from build123d import *

# Parameters (mm, degrees)
BOSS_EXTRUDE1_DEPTH            = 3
SKETCH2_R                      = 2
CUT_EXTRUDE1_DEPTH             = 3
CHAMFER1_SIZE                  = 0.5
LPATTERN1_COUNT                = 14
LPATTERN1_PITCH                = 50
CHAMFER1_OF_LPATTERN1_SIZE     = 0.5
LPATTERN1_COL_COUNT            = 14
LPATTERN1_COL_PITCH            = 50
CHAMFER1_OF_LPATTERN1_COL_SIZE = 0.5
FILLET1_R                      = 1
SKETCH3_R                      = 2.25
CUT_EXTRUDE2_DEPTH             = 10
CHAMFER2_SIZE                  = 0.5
CHAMFER2_OF_MIRROR1_SIZE       = 0.5


with BuildPart() as part:
    # Sketch1 → Boss-Extrude1 (new body)
    with BuildSketch(Plane(origin=(0, 0, 0), x_dir=(0, 0, -1), z_dir=(1, 0, 0))):
        Polygon((-706, 30), (-706, -5), (-671, -5), (-671, -30), (671, -30), (671, -5), (706, -5), (706, 30), align=None)
    extrude(amount=BOSS_EXTRUDE1_DEPTH)

    # Sketch2 → Cut-Extrude1 (cut)
    with BuildSketch(Plane(origin=(3, 0, 0), x_dir=(0, 0, -1), z_dir=(1, 0, 0))):
        with Locations((0, -25)):
            Circle(SKETCH2_R)
    cut_extrude1 = extrude(amount=-CUT_EXTRUDE1_DEPTH, mode=Mode.SUBTRACT)

    # Chamfer1
    chamfer1_edges = [part.edges().sort_by_distance(p)[0] for p in [
        (3, -25, 2),
    ]]
    chamfer(chamfer1_edges, length=CHAMFER1_SIZE)

    # LPattern1: Cut-Extrude1 ×14
    with Locations(*[(0, 0, i * LPATTERN1_PITCH) for i in range(1, LPATTERN1_COUNT)]):
        add(cut_extrude1, mode=Mode.SUBTRACT)

    # Chamfer1 of LPattern1
    chamfer1_of_lpattern1_edges = [part.edges().sort_by_distance(p)[0] for p in [
        (3, -25, 52),
        (3, -25, 102),
        (3, -25, 152),
        (3, -25, 202),
        (3, -25, 252),
        (3, -25, 302),
        (3, -25, 352),
        (3, -25, 402),
        (3, -25, 452),
        (3, -25, 502),
        (3, -25, 552),
        (3, -25, 602),
        (3, -25, 652),
    ]]
    chamfer(chamfer1_of_lpattern1_edges, length=CHAMFER1_OF_LPATTERN1_SIZE)

    # LPattern1 col: Cut-Extrude1 ×14
    with Locations(*[(0, 0, -i * LPATTERN1_COL_PITCH) for i in range(1, LPATTERN1_COL_COUNT)]):
        add(cut_extrude1, mode=Mode.SUBTRACT)

    # Chamfer1 of LPattern1 col
    chamfer1_of_lpattern1_col_edges = [part.edges().sort_by_distance(p)[0] for p in [
        (3, -25, -48),
        (3, -25, -98),
        (3, -25, -148),
        (3, -25, -198),
        (3, -25, -248),
        (3, -25, -298),
        (3, -25, -348),
        (3, -25, -398),
        (3, -25, -448),
        (3, -25, -498),
        (3, -25, -548),
        (3, -25, -598),
        (3, -25, -648),
    ]]
    chamfer(chamfer1_of_lpattern1_col_edges, length=CHAMFER1_OF_LPATTERN1_COL_SIZE)

    # Fillet1
    fillet1_edges = [part.edges().sort_by_distance(p)[0] for p in [
        (1.5, -5, -706),
        (1.5, -30, -671),
        (1.5, -30, 671),
        (1.5, -5, 706),
        (1.5, 30, 706),
        (1.5, 30, -706),
    ]]
    fillet(fillet1_edges, radius=FILLET1_R)

    # Sketch3 → Cut-Extrude2 (cut)
    with BuildSketch(Plane(origin=(3, 0, 0), x_dir=(0, 0, -1), z_dir=(1, 0, 0))):
        with Locations((687, 12)):
            Circle(SKETCH3_R)
    cut_extrude2 = extrude(amount=-CUT_EXTRUDE2_DEPTH, mode=Mode.SUBTRACT)

    # Chamfer2
    chamfer2_edges = [part.edges().sort_by_distance(p)[0] for p in [
        (3, 12, -684.75),
    ]]
    chamfer(chamfer2_edges, length=CHAMFER2_SIZE)

    # Mirror1: Cut-Extrude2 across plane
    add(cut_extrude2.mirror(Plane.XY), mode=Mode.SUBTRACT)

    # Chamfer2 of Mirror1
    chamfer2_of_mirror1_edges = [part.edges().sort_by_distance(p)[0] for p in [
        (3, 12, 684.75),
    ]]
    chamfer(chamfer2_of_mirror1_edges, length=CHAMFER2_OF_MIRROR1_SIZE)


solid = part.part
Source: CAD feature listing. Evaluate the final solid. Frame: model axes, mm. Round coordinates to 2 decimals unless told otherwise and drop trailing zeros.
Q1. Ray query, line 1 (Z direction, x = 2.5, y = 13); line 2 (Y direction, x = 1.5, z = 687); line 3 (Y direction, x = 1.25, z = 300). Return the intervals inside material, ascending.
Q2. Section A-A, the plane x = 1.5. State how many separate pieces and enclosed holes the cut face has, plus the area to 3 significant figures.
Q3. First-contact query: P1, Ø3.5, axis at y = -25, z = 600, coming from the +X side; P2, Ø4.5, axis at y = -25, z = -100, coming from the +X side. Flat tips, straight axial feed; report the tip coordinate or a pass-through.
Solutions:
1. line 1: z = -706 to -689.02, -684.98 to 684.98, 689.02 to 706
1. line 2: y = -5 to 9.75, 14.25 to 30
1. line 3: y = -30 to -27, -23 to 30
2. separate pieces: 1
2. enclosed holes: 29
2. area: 82,600 mm2
3. P1: passes through
3. P2: stops at x = 2.75
